Check sheet for the modelled part. Datum: model origin and axes. Units: mm. A direction names the side the tool comes from. Give positions to 0.01 mm unless a question says otherwise; leave off trailing zeros. Write each loop counter-clockwise with the first axis right and the second up, starting at its lowest first coordinate (ties: lowest second). Pieces come first, ordered by that corner, then holes. Notation, with made-up numbers: M 53.5,17 L 102.5,17 A22 cw 102.5,48 Z; hole C -7.75,-31.5 d11. An arc over 180 degrees is marked long. Write item = value, one per line. Start each with the question number.
1) Scan lines: L1, parallel to Y at x = -83, z = 0.7; L2, parallel to Y at x = -66.5, z = 4.8; L3, parallel to Y at x = -63.5, z = 3.65. Record each from-to range of solid material in increasing order.
2) Gauge pin test, flat ends, axial feed: pin 1 (2.5 mm diameter, centred on x = -93.5, z = 3, fed in from -Y); pin 2 (4 mm diameter, centred on x = -71, y = 9, fed in from -Z); pin 3 (1.5 mm diameter, centred on x = -39, z = 0.5, fed in from -Y); pin 4 (2.5 mm diameter, centred on y = -102, z = 3, fed in from -X). Record the tip position at first contact, or that the pin passes through.
3) Sectioned sample at D-D, the plane y = 94.5. Record the cut outline in (x, z).
4) Sectioned sample at C-C, the plane y = -73. Record the cut outline in (x, z).
5) Sectioned sample at B-B, the plane z = 4.15. Record the cut outline in (x, y).
6) Set-up check for faces 1 (the face through (-66, 2, 0)), 2 (the face through (-55.81, -71.39, 2.54)), 3 (the face through (-90, -91.5, 3)): record each of +Z, -Z, +X, -X, +Y, -Y from which the full face is reachable in a straight line by a thin tool's end or side.
7) Sectioned sample at A-A, the plane x = -63. Record the cut outline in (y, z), then the cut area to 3 significant figures.
from build123d import *

# Parameters (mm, degrees)
SKETCH1_W           = 200
SKETCH1_H           = 225
BOSS_EXTRUDE1_DEPTH = 5
SKETCH2_W           = 21
SKETCH2_H           = 21
CUT_EXTRUDE1_DEPTH  = 151.602954818
CUT_EXTRUDE2_DEPTH  = 151.602954818


with BuildPart() as part:
    # Sketch1 → Boss-Extrude1 (new body)
    with BuildSketch(Plane.XY):
        Rectangle(SKETCH1_W, SKETCH1_H)
    extrude(amount=BOSS_EXTRUDE1_DEPTH)

    # Sketch2 → Cut-Extrude1 (cut, through all)
    with BuildSketch(Plane.XY.offset(5)):
        with Locations((-89.5, -102)):
            Rectangle(SKETCH2_W, SKETCH2_H)
    extrude(amount=-CUT_EXTRUDE1_DEPTH, mode=Mode.SUBTRACT)

    # Sketch3 → Cut-Extrude2 (cut, through all)
    with BuildSketch(Plane.XY.offset(5)):
        Polygon((-47.115076642, -95.712122393), (-48.11426359, -112.5), (100, -112.5), (100, 112.5), (-41.68901441, 112.5), (-31.902672347, 30.754430855), (-36.262952178, -42.504976974), (-67.144755679, -49.596294754), (-44.155064893, -93.798693152), align=None)
    extrude(amount=-CUT_EXTRUDE2_DEPTH, mode=Mode.SUBTRACT)


solid = part.part
Data:
q1.L1 = -91.5 to 112.5
q1.L2 = -112.5 to -50.84, -49.45 to 112.5
q1.L3 = -112.5 to -56.6, -48.76 to 112.5
q2.pin_1 = -91.5
q2.pin_2 = 0
q2.pin_3 = -43.31
q2.pin_4 = -79
q3.outline = M -100,0 L -39.53,0 L -39.53,5 L -100,5 Z
q4.outline = M -100,0 L -54.97,0 L -54.97,5 L -100,5 Z
q5.outline = M -100,-91.5 L -79,-91.5 L -79,-112.5 L -48.11,-112.5 L -47.12,-95.71 L -44.16,-93.8 L -67.14,-49.6 L -36.26,-42.5 L -31.9,30.75 L -41.69,112.5 L -100,112.5 Z
q6.face_1 = -Z, +X, -X, +Y, -Y
q6.face_2 = +Z, -Z, +X
q6.face_3 = +Z, -Z, -X, -Y
q7.outline = M -112.5,0 L -57.57,0 L -57.57,5 L -112.5,5 Z; M -48.64,0 L 112.5,0 L 112.5,5 L -48.64,5 Z
q7.area = 1,080 mm2
